Could you check a few things on this model? Use its own coordinates, in mm. A direction names the side the tool comes from. Give positions to 0.01 mm unless a question says otherwise; leave off trailing zeros. Order: outer loops, then holes, each group sorted by start corner. A loop starts at its lowest first (then second) coordinate and runs counter-clockwise, first axis right, second up. Notation, with made-up numbers: M -6.75,-21.75 L 41.25,-21.75 A15 cw 41.25,3.25 Z; hole C 52,-4.5 d8. An arc over 180 degrees is marked long. Use a Markdown table: item, result. Add a question column.
Item 1: Suppose I cut it at C-C on y = -24. Write out the boundary of the cut face in (x, z).
Item 2: For faces 1 (the face through (-61.2, -6.2, -53)), 2 (the face through (1, -10, -55)), 3 (the face through (1, -35, -53)), which set-ups out of +Z, -Z, +X, -X, +Y, -Y let a thin tool reach every point of the face, with its end or its side?
Item 3: If we mould it in two halves opening along X, with no side actions, what happens to faces 4 (the face through (-55, -20, -56)), 5 (the face through (-66.161, -35, -55)), 6 (the face through (-30, -20, -3)), 7 (the face through (5.839, -35, -55))? For each: released by +X, released by -X, zero draft, split by the parting line, or undercut.
Item 4: If I drill on L1, parallel to X at y = -35, z = -55; L2, parallel to X at y = -15.5, z = -18; L3, parallel to Z at x = -34.5, y = -3, over which ranges is the centre line in solid material (lowest first)? Write a range as from..to.
Item 5: Suppose I cut it at D-D on x = -51.5. Write out the boundary of the cut face in (y, z).
Item 6: Suppose I cut it at B-B on y = -35. Write out the boundary of the cut face in (x, z), plus the area to 3 significant figures.
Item 7: Suppose I cut it at A-A on z = -12.5. Write out the boundary of the cut face in (x, y).
Item 8: I'm going to push flat-ended pins straight in: pin 1 Ø5 at (y, z) = (-21.5, -17) entering from -X; pin 2 Ø2 at (y, z) = (-14, -9) entering from +X; pin 3 Ø5 at (x, y) = (-63, -36) entering from +Z. Where does each tip first touch, or does it pass through?
from build123d import *

# Parameters (mm, degrees)
F1_DEPTH = 40
F3_W     = 10
F3_H     = 10
F4_DEPTH = 3
F2_W     = 10
F2_H     = 10
F5_DEPTH = 3
F6_W     = 10
F6_H     = 10
F7_DEPTH = 3
F8_W     = 10
F8_H     = 10
F9_DEPTH = 3
F11_D    = 3


# Not quite as in the source:
# - a feature of the source that left no trace in its solid (it failed there, or was rolled back) is left out
# - a feature names something its author has since deleted; it is built from what else it names


with BuildPart() as f1:
    # F0 (on Front) → F1 (new body)
    with BuildSketch(Plane.XZ):
        Polygon((-56.1606403851, 0), (-56.1606403851, -56), (-53.1606403851, -56), (-53.1606403851, -3), (-7.1606403851, -3), (-7.1606403851, -56), (-4.1606403851, -56), (-4.1606403851, 0), align=None)
    extrude(amount=F1_DEPTH)

    # F3 (on face) → F4 (join)
    with BuildSketch(Plane(origin=(0, 0, -56), x_dir=(1, 0, 0), z_dir=(0, 0, -1))):
        with Locations((0.8393596149, 5)):
            Rectangle(F3_W, F3_H)
    extrude(amount=-F4_DEPTH)

    # F2 (on face) → F5 (join)
    with BuildSketch(Plane(origin=(0, 0, -56), x_dir=(1, 0, 0), z_dir=(0, 0, -1))):
        with Locations((-61.1606403851, 5)):
            Rectangle(F2_W, F2_H)
    extrude(amount=-F5_DEPTH)

    # F6 (on face) → F7 (join)
    with BuildSketch(Plane(origin=(0, 0, -56), x_dir=(1, 0, 0), z_dir=(0, 0, -1))):
        with Locations((0.8393596149, 35)):
            Rectangle(F6_W, F6_H)
    extrude(amount=-F7_DEPTH)

    # F8 (on face) → F9 (join)
    with BuildSketch(Plane(origin=(0, 0, -56), x_dir=(1, 0, 0), z_dir=(0, 0, -1))):
        with Locations((-61.1606403851, 35)):
            Rectangle(F8_W, F8_H)
    extrude(amount=-F9_DEPTH)

    # F11 (through all)
    with Locations(Plane(origin=(0, 0, -56), x_dir=(1, 0, 0), z_dir=(0, 0, -1))):
        with Locations((-61.6680905223, 35), (18.8430529088, 95.1308980584), (-61.3079555333, 4.5014377683), (19.3945541978, 4.6852682717)):
            Hole(F11_D / 2)


solid = f1.part
Findings below:
| question | item | result |
|---|---|---|
| 1 | outline | M -56.16,-56 L -53.16,-56 L -53.16,-3 L -7.16,-3 L -7.16,-56 L -4.16,-56 L -4.16,0 L -56.16,0 Z |
| 2 | face 1 | +Z, -X, +Y, -Y |
| 2 | face 2 | +Z, -Z, +X |
| 2 | face 3 | +Z, +X, +Y, -Y |
| 3 | face 4 | zero draft |
| 3 | face 5 | released by -X |
| 3 | face 6 | undercut |
| 3 | face 7 | released by +X |
| 4 | L1 | x = -66.16..-63.17, -60.17..-53.16, -7.16..5.84 |
| 4 | L2 | x = -56.16..-53.16, -7.16..-4.16 |
| 4 | L3 | z = -3..0 |
| 5 | outline | M -40,-3 L 0,-3 L 0,0 L -40,0 Z |
| 6 | outline | M -66.16,-56 L -63.17,-56 L -63.17,-53 L -66.16,-53 Z; M -60.17,-56 L -53.16,-56 L -53.16,-3 L -7.16,-3 L -7.16,-56 L 5.84,-56 L 5.84,-53 L -4.16,-53 L -4.16,0 L -56.16,0 L -56.16,-53 L -60.17,-53 Z |
| 6 | area | 525 mm^2 |
| 7 | outline | M -56.16,-40 L -53.16,-40 L -53.16,0 L -56.16,0 Z; M -7.16,-40 L -4.16,-40 L -4.16,0 L -7.16,0 Z |
| 8 | pin 1 | stops at x = -56.16 |
| 8 | pin 2 | stops at x = -4.16 |
| 8 | pin 3 | stops at z = -53 |
